Can you work these out from the model? Positions are in its coordinate system, mm. Round coordinates to 2 decimals unless told otherwise and drop trailing zeros. Loops run counter-clockwise (first coordinate to the right, second up) from the corner with the lowest first, then second, coordinate; pieces in that order, holes last.
from build123d import *

# Parameters (mm, degrees)
BOSS_EXTRUDE1_DEPTH = 3
FILLET1_R           = 40


with BuildPart() as part:
    # Sketch1 → Boss-Extrude1 (new body)
    with BuildSketch(Plane.XY):
        Polygon((0, 0), (0, 100), (223.5, 100), (223.5, 85), (226.5, 85), (226.5, 100), (450, 100), (450, 0), (420, 0), (420, 70), (275, 70), (260, 65), (190, 65), (175, 70), (30, 70), (30, 0), align=None)
    extrude(amount=BOSS_EXTRUDE1_DEPTH)

    # Fillet1
    fillet1_edges = [part.edges().sort_by_distance(p)[0] for p in [
        (420, 70, 1.5),
        (275, 70, 1.5),
        (260, 65, 1.5),
        (190, 65, 1.5),
        (175, 70, 1.5),
        (30, 70, 1.5),
    ]]
    fillet(fillet1_edges, radius=FILLET1_R)


solid = part.part
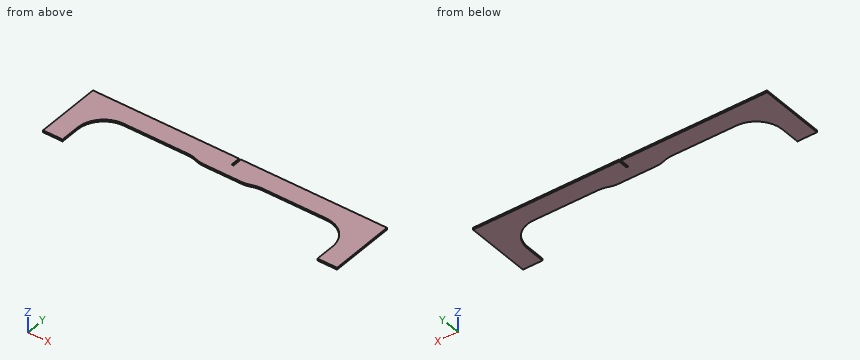
(1) Will these pins go through, and if not, where does the flat tip stop? P1, Ø0.9, axis at x = 224.5, z = 1, coming from the -Y side; P2, Ø1.5, axis at x = 106, z = 2, coming from the -Y side.
Worked answers:
P1: stops at y = 65
P2: stops at y = 70
(2) If we section it at A-A, the plane y = 12: List the corners of the cut face in (x, z) for me, then the cut area to 3 significant figures.
Worked answers:
outline: (0, 0) - (30, 0) - (30, 3) - (0, 3) - close; (420, 0) - (450, 0) - (450, 3) - (420, 3) - close
area: 180 mm2
(3) If we section it at C-C, the plane x = 215: List the corners of the cut face in (y, z) for me.
Worked answers:
outline: (65, 0) - (100, 0) - (100, 3) - (65, 3) - close
(4) If we section it at D-D, the plane y = 37.5: List the corners of the cut face in (x, z) for me.
Worked answers:
outline: (0, 0) - (30.71, 0) - (30.71, 3) - (0, 3) - close; (419.29, 0) - (450, 0) - (450, 3) - (419.29, 3) - close
(5) If I drill on line 1 (X direction, y = 18, z = 1.55); line 2 (X direction, y = 88, z = 1.25); line 3 (Y direction, x = 197, z = 2.3), over which ranges is the centre line in solid material (lowest first)?
Worked answers:
line 1: x = 0 to 30, 420 to 450
line 2: x = 0 to 223.5, 226.5 to 450
line 3: y = 65 to 100
(6) If we section it at B-B, the plane z = 1.2: List the corners of the cut face in (x, y) for me, then the cut area to 3 significant figures.
Worked answers:
outline: (0, 0) - (30, 0) - (30, 30) arc R40 cw to (70, 70) - (168.51, 70) arc R40 cw to (181.16, 67.95) - (183.84, 67.05) arc R40 ccw to (196.49, 65) - (253.51, 65) arc R40 ccw to (266.16, 67.05) - (268.84, 67.95) arc R40 cw to (281.49, 70) - (380, 70) arc R40 cw to (420, 30) - (420, 0) - (450, 0) - (450, 100) - (226.5, 100) - (226.5, 85) - (223.5, 85) - (223.5, 100) - (0, 100) - close
area: 18,800 mm2
